```python
from build123d import *

# Parameters (mm, degrees)
SKETCH_W          = 220
SKETCH_H          = 180
PAD_DEPTH         = 10
BOX_W             = 220
BOX_H             = 3
BOX_DEPTH         = 3
FILLET_R          = 1
CYLINDER_R        = 17
CYLINDER_DEPTH    = 40
CYLINDER001_R     = 16
CYLINDER001_DEPTH = 40
CYLINDER002_R     = 17
CYLINDER002_DEPTH = 40
CYLINDER003_R     = 17
CYLINDER003_DEPTH = 40
CYLINDER004_R     = 17
CYLINDER004_DEPTH = 40
CYLINDER005_R     = 17
CYLINDER005_DEPTH = 40
CYLINDER006_R     = 16
CYLINDER006_DEPTH = 40
CYLINDER007_R     = 16
CYLINDER007_DEPTH = 40
CYLINDER008_R     = 16
CYLINDER008_DEPTH = 40
CYLINDER009_R     = 16
CYLINDER009_DEPTH = 40
CYLINDER012_R     = 38
CYLINDER012_DEPTH = 40
CYLINDER013_R     = 37
CYLINDER013_DEPTH = 40


with BuildPart() as part:
    # Sketch → Pad (new body)
    with BuildSketch(Plane.XY):
        with Locations((20.312759, 0)):
            Rectangle(SKETCH_W, SKETCH_H)
    extrude(amount=PAD_DEPTH)

    # Box → Box (join)
    with BuildSketch(Plane(origin=(-90, -93, 3), x_dir=(1, 0, 0), z_dir=(0, 0, 1))):
        with Locations((110, 1.5)):
            Rectangle(BOX_W, BOX_H)
    extrude(amount=BOX_DEPTH)

    # Fillet
    fillet_edges = [part.edges().sort_by_distance(p)[0] for p in [
        (20, -93, 3),
        (130, -93, 4.5),
        (20, -93, 6),
        (-90, -93, 4.5),
    ]]
    fillet(fillet_edges, radius=FILLET_R)

    # Cylinder → Cylinder (join)
    with BuildSketch(Plane(origin=(-60, -65, 10), x_dir=(1, 0, 0), z_dir=(0, 0, 1))):
        Circle(CYLINDER_R)
    extrude(amount=CYLINDER_DEPTH)

    # Cylinder001 → Cylinder001 (cut)
    with BuildSketch(Plane(origin=(-60, -65, 10), x_dir=(1, 0, 0), z_dir=(0, 0, 1))):
        Circle(CYLINDER001_R)
    extrude(amount=CYLINDER001_DEPTH, mode=Mode.SUBTRACT)

    # Cylinder002 → Cylinder002 (join)
    with BuildSketch(Plane(origin=(-20, -65, 10), x_dir=(1, 0, 0), z_dir=(0, 0, 1))):
        Circle(CYLINDER002_R)
    extrude(amount=CYLINDER002_DEPTH)

    # Cylinder003 → Cylinder003 (join)
    with BuildSketch(Plane(origin=(20, -65, 10), x_dir=(1, 0, 0), z_dir=(0, 0, 1))):
        Circle(CYLINDER003_R)
    extrude(amount=CYLINDER003_DEPTH)

    # Cylinder004 → Cylinder004 (join)
    with BuildSketch(Plane(origin=(60, -65, 10), x_dir=(1, 0, 0), z_dir=(0, 0, 1))):
        Circle(CYLINDER004_R)
    extrude(amount=CYLINDER004_DEPTH)

    # Cylinder005 → Cylinder005 (join)
    with BuildSketch(Plane(origin=(100, -65, 10), x_dir=(1, 0, 0), z_dir=(0, 0, 1))):
        Circle(CYLINDER005_R)
    extrude(amount=CYLINDER005_DEPTH)

    # Cylinder006 → Cylinder006 (cut)
    with BuildSketch(Plane(origin=(-20, -65, 10), x_dir=(1, 0, 0), z_dir=(0, 0, 1))):
        Circle(CYLINDER006_R)
    extrude(amount=CYLINDER006_DEPTH, mode=Mode.SUBTRACT)

    # Cylinder007 → Cylinder007 (cut)
    with BuildSketch(Plane(origin=(20, -65, 10), x_dir=(1, 0, 0), z_dir=(0, 0, 1))):
        Circle(CYLINDER007_R)
    extrude(amount=CYLINDER007_DEPTH, mode=Mode.SUBTRACT)

    # Cylinder008 → Cylinder008 (cut)
    with BuildSketch(Plane(origin=(60, -65, 10), x_dir=(1, 0, 0), z_dir=(0, 0, 1))):
        Circle(CYLINDER008_R)
    extrude(amount=CYLINDER008_DEPTH, mode=Mode.SUBTRACT)

    # Cylinder009 → Cylinder009 (cut)
    with BuildSketch(Plane(origin=(100, -65, 10), x_dir=(1, 0, 0), z_dir=(0, 0, 1))):
        Circle(CYLINDER009_R)
    extrude(amount=CYLINDER009_DEPTH, mode=Mode.SUBTRACT)

    # Cylinder012 → Cylinder012 (join)
    with BuildSketch(Plane(origin=(-40, -5, 10), x_dir=(1, 0, 0), z_dir=(0, 0, 1))):
        Circle(CYLINDER012_R)
    extrude(amount=CYLINDER012_DEPTH)

    # Cylinder013 → Cylinder013 (cut)
    with BuildSketch(Plane(origin=(-40, -5, 10), x_dir=(1, 0, 0), z_dir=(0, 0, 1))):
        Circle(CYLINDER013_R)
    extrude(amount=CYLINDER013_DEPTH, mode=Mode.SUBTRACT)


solid = part.part
```
The listing builds one solid part. Answer for the finished solid, in the listing's coordinates (mm). A direction names the side the tool comes from. Coordinates: 2 decimals unless noted, no trailing zeros. Write each loop counter-clockwise with the first axis right and the second up, starting at its lowest first coordinate (ties: lowest second). Pieces come first, ordered by that corner, then holes.
Q1. Section C-C, the plane x = 60 is taken. Write down the section's boundary in (y, z), then the cut area to 3 significant figures.
Returned:
outline: (-93, 4) arc R1 ccw to (-92, 3) - (-90, 3) - (-90, 0) - (90, 0) - (90, 10) - (-48, 10) - (-48, 50) - (-49, 50) - (-49, 10) - (-81, 10) - (-81, 50) - (-82, 50) - (-82, 10) - (-90, 10) - (-90, 6) - (-92, 6) arc R1 ccw to (-93, 5) - close
area: 1,890 mm2
Q2. Section D-D, the plane y = -25.5 is taken. Write down the section's boundary in (x, z).
Returned:
outline: (-89.69, 0) - (130.31, 0) - (130.31, 10) - (-8, 10) - (-8, 50) - (-9.2, 50) - (-9.2, 10) - (-70.8, 10) - (-70.8, 50) - (-72, 50) - (-72, 10) - (-89.69, 10) - close
Q3. Given P1, Ø6, axis at y = 18, z = 41.5, coming from the -X side; P2, Ø11, axis at y = 29.5, z = 3.5, coming from the -X side; P3, Ø1.6, axis at x = 44.5, y = -91.5, coming from the +Z side; P4, Ø1.5, axis at y = 34.5, z = 27, coming from the +X side, each flat-ended and moving along its own axis, determine where each tip first touches the part or whether it passes through.
Returned:
P1: stops at x = -72.31
P2: stops at x = -89.69
P3: stops at z = 6
P4: passes through
Q4. Which of the six approach directions +Z, -Z, +X, -X, +Y, -Y give full straight-line access (tool end or side, diameter ignored) to faces 5 (the cylindrical face through (-75.985, -64.297, 29.72)), 6 (the flat face through (70, -78, 50))?
Returned:
face 5: +Z
face 6: +Z, +X, -X, +Y, -Y
Q5. Section B-B, the plane y = -5 is taken. Write down the section's boundary in (x, z).
Returned:
outline: (-89.69, 0) - (130.31, 0) - (130.31, 10) - (-2, 10) - (-2, 50) - (-3, 50) - (-3, 10) - (-77, 10) - (-77, 50) - (-78, 50) - (-78, 10) - (-89.69, 10) - close
Q6. Section A-A, the plane z = 30.5 is taken. Give the number of separate pieces and of enclosed holes in the cut face, then the cut area to 3 significant figures.
Returned:
separate pieces: 6
enclosed holes: 6
area: 754 mm2
Q7. The mould has two halves that part along Y. Classify faces 1 (the flat face through (19, 90, 5)), 2 (the flat face through (-41, -4, 10)), 3 (the cylindrical face through (16.315, -81.596, 29.72)), 4 (the flat face through (-7, -75, 50)): released by +Y, released by -Y, zero draft, split by the parting line, or undercut.
Returned:
face 1: released by +Y
face 2: undercut
face 3: split by the parting line
face 4: zero draft
Q8. Find the intervals of material crossed by line 1 along Y through (x, z) = (-40, 22); line 2 along Y through (x, z) = (19, 28.5); line 3 along X through (y, z) = (-3, 15), in increasing order.
Returned:
line 1: y = -43 to -42, 32 to 33
line 2: y = -81.97 to -80.97, -49.03 to -48.03
line 3: x = -77.95 to -76.95, -3.05 to -2.05
